Input: part model. Units: mm. Frame: model coordinates. Face numbers are marked on the shaded views. Coordinates: 2 decimals unless noted, no trailing zeros. Order: outer loops, then holes, each group sorted by start corner. A loop starts at its lowest first (then second) coordinate and runs counter-clockwise, first axis right, second up.
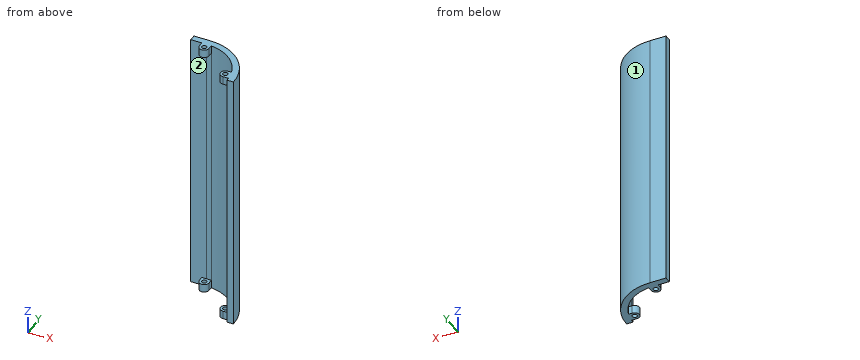
from build123d import *

# Parameters (mm, degrees)
SKETCH_1_R          = 1.5
EXTRUDE_1_DEPTH     = 162
CUT_EXTRUDE_1_DEPTH = 76


with BuildPart() as part:
    # 草图1 → 凸台-拉伸1 (new body)
    with BuildSketch(Plane.XY):
        with BuildLine():
            Line((-6.315789474, 9.394736842), (-6.315789474, 12.394736842))
            Line((-6.315789474, 12.394736842), (-13.315789474, 12.394736842))
            Line((-13.315789474, 12.394736842), (-13.315789474, 16.394736842))
            Line((-13.315789474, 16.394736842), (-3.315789474, 16.394736842))
            ThreePointArc((-3.315789474, 16.394736842), (17.897413962, 7.607940278), (26.684210526, -13.605263158))
            Line((26.684210526, -13.605263158), (22.684210526, -13.605263158))
            ThreePointArc((22.684210526, -13.605263158), (22.664944086, -12.604521591), (22.60717332, -11.605263158))
            Line((22.60717332, -11.605263158), (19.134154847, -11.605263158))
            ThreePointArc((19.134154847, -11.605263158), (16.134154847, -8.605263158), (19.134154847, -5.605263158))
            Line((19.134154847, -5.605263158), (21.42284428, -5.605263158))
            ThreePointArc((21.42284428, -5.605263158), (13.170646711, 6.499398539), (-0.315789474, 12.221079982))
            Line((-0.315789474, 12.221079982), (-0.315789474, 9.394736842))
            ThreePointArc((-0.315789474, 9.394736842), (-3.315789474, 6.394736842), (-6.315789474, 9.394736842))
        make_face()
        with Locations((-3.315789474, 9.394736842)):
            Circle(SKETCH_1_R, mode=Mode.SUBTRACT)
        with Locations((19.134154847, -8.605263158)):
            Circle(SKETCH_1_R, mode=Mode.SUBTRACT)
    extrude(amount=EXTRUDE_1_DEPTH)

    # 草图3 → 切除-拉伸1 (cut, symmetric)
    with BuildSketch(Plane.XY.offset(81)):
        with BuildLine():
            Line((-3.315789474, 12.394736842), (-13.315789474, 12.394736842))
            Line((-13.315789474, 12.394736842), (-18.728718327, 7.33373453))
            ThreePointArc((-18.728718327, 7.33373453), (4.795500809, -38.307630857), (-3.315789474, 12.394736842))
        make_face()
    extrude(amount=CUT_EXTRUDE_1_DEPTH, both=True, mode=Mode.SUBTRACT)


solid = part.part
Item 1: Cut plane C-C on y = 3. Return loops of the section in (x, z).
Response values:
outline: (16.69, 0) - (21.67, 0) - (21.67, 162) - (16.69, 162) - close
Item 2: Pin query (flat end, axial travel): pin 1 Ø3 at (x, y) = (19.5, -8) entering from +Z; pin 2 Ø8 at (y, z) = (-8.5, 27) entering from -X; pin 3 Ø1 at (y, z) = (2, 112) entering from -X; pin 4 Ø1.1 at (x, z) = (19.5, 159) entering from +Y. Return the tip coordinate at first contact, or that it passes through.
Response values:
pin 1: stops at z = 162
pin 2: stops at x = 21.04
pin 3: stops at x = 17.1
pin 4: stops at y = 6.5
Item 3: Cut plane A-A on z = 141. Return loops of the section in (x, y).
Response values:
outline: (-13.32, 12.39) - (-3.32, 12.39) arc R26 cw to (22.68, -13.61) - (26.68, -13.61) arc R30 ccw to (-3.32, 16.39) - (-13.32, 16.39) - close
Item 4: Draft query along Z for the marked faces 1 and 2. Return one class per face: pulls with the +Z half, pulls with the -Z half, needs draft (parallel to the pull), parting line crosses it, or undercut.
Response values:
face 1: needs draft
face 2: undercut
Item 5: Ray query, probe 1 along Y at (x, z) = (-10, 66.5); probe 2 along X at (y, z) = (-7.5, 80.5); probe 3 along X at (y, z) = (1.5, 29.5). Return the intervals inside material, ascending.
Response values:
probe 1: y = 12.39 to 16.39
probe 2: x = 21.96 to 26.06
probe 3: x = 17.85 to 22.6
Item 6: Cut plane B-B on x = -10. Return loops of the section in (y, z), then the cut area to 3 significant figures.
Response values:
outline: (12.39, 0) - (16.39, 0) - (16.39, 162) - (12.39, 162) - close
area: 648 mm2
